Verification items for this drawing (mm, ordinates from the low corner). Coordinates: 2 decimals unless noted, no trailing zeros. Order: outer loops, then holes, each group sorted by start corner. A loop starts at its lowest first (then second) coordinate and runs counter-clockwise, first axis right, second up. Notation, with made-up numbers: (42.25, 52) -> (49.25, 52) arc R19 cw to (49.25, 62) -> close; hole circle Ø9 at (9.25, -4.5). An arc over 180 degrees is marked (long way). Answer as CSV lines item,"result". Start each with the question number.
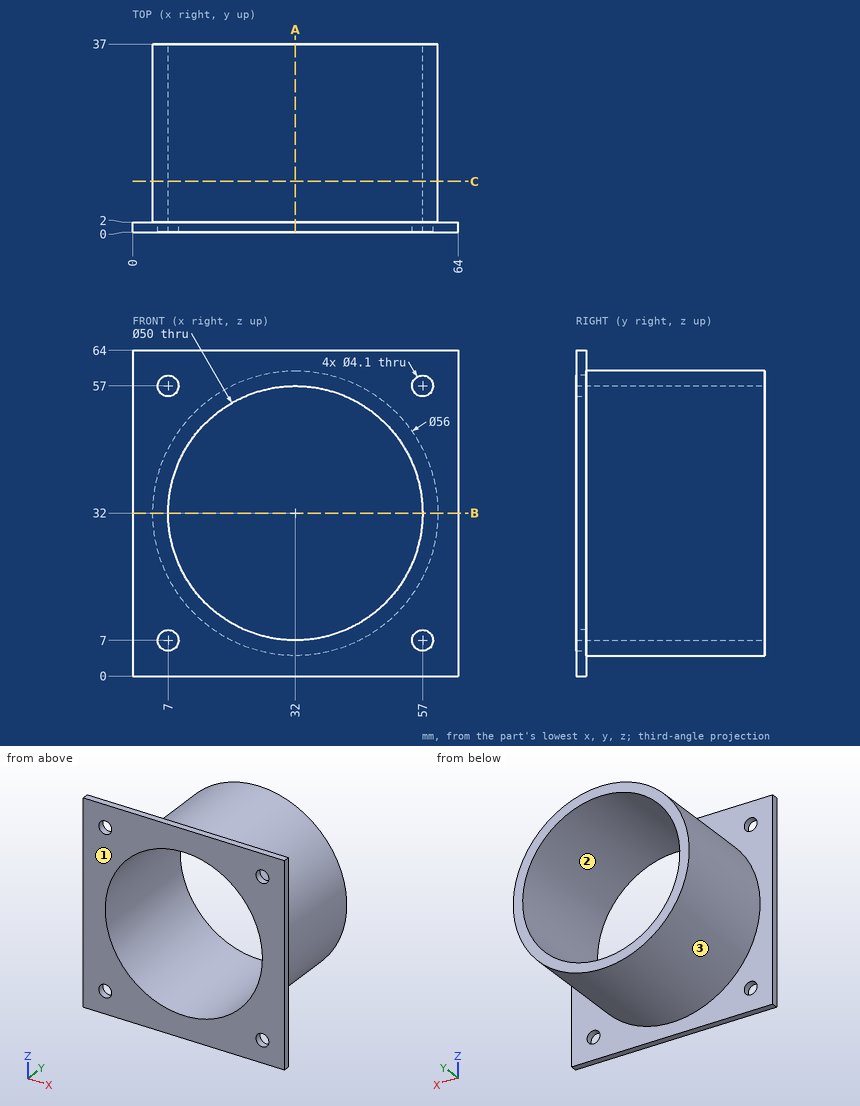
Q1. Thickness scan on L1, parallel to Z at x = 31.5, y = 9.5 (3 decimals); L2, parallel to Z at x = 23, y = 27; L3, parallel to X at y = 30, z = 17. Record the ranges inside material, lowest first.
Q2. Sectioned sample at B-B, the plane z = 32. Record the cut outline in (x, y).
Q3. Sectioned sample at C-C, the plane y = 10. Record the cut outline in (x, z).
Q4. Release check for a two-part mould opening along Z. For the marked faces 1, 2 and 3 record: released by +Z, released by -Z, zero draft, split by the parting line, or undercut.
Q5. Sectioned sample at A-A, the plane x = 32. Record the cut outline in (y, z), then the cut area to 3 significant figures.
Q6. Go/stop test with flat-tipped pins: pin 1 Ø3 at (x, y) = (56, 12) entering from +Z; pin 2 Ø12 at (x, y) = (16, 22) entering from -Z; pin 3 Ø5.5 at (x, z) = (7, 57) entering from +Y. Record where each tip stops, or that it passes through.
Geometry results:
1,L1,"z = 4.004 to 7.005, 56.995 to 59.996"
1,L2,"z = 5.49 to 8.68, 55.32 to 58.51"
1,L3,"x = 8.36 to 12, 52 to 55.64"
2,outline,"(0, 0) -> (7, 0) -> (7, 37) -> (4, 37) -> (4, 2) -> (0, 2) -> close; (57, 0) -> (64, 0) -> (64, 2) -> (60, 2) -> (60, 37) -> (57, 37) -> close"
3,outline,"circle Ø56 at (32, 32); hole circle Ø50 at (32, 32)"
4,face 1,"zero draft"
4,face 2,"undercut"
4,face 3,"split by the parting line"
5,outline,"(0, 0) -> (2, 0) -> (2, 4) -> (37, 4) -> (37, 7) -> (0, 7) -> close; (0, 57) -> (37, 57) -> (37, 60) -> (2, 60) -> (2, 64) -> (0, 64) -> close"
5,area,"238 mm^2"
6,pin 1,"stops at z = 48.67"
6,pin 2,"stops at z = 5.85"
6,pin 3,"stops at y = 2"
